Design review of the part built by this model. Coordinates are the model's own, in mm. A direction names the side the tool comes from. Give positions to 0.01 mm unless a question says otherwise; leave off trailing zeros. Loops run counter-clockwise (first coordinate to the right, second up) from the corner with the lowest first, then second, coordinate; pieces in that order, holes last.
from build123d import *

# Parameters (mm, degrees)
SKETCH_1_W          = 106
SKETCH_1_H          = 103
SKETCH_1_W_2        = 102
SKETCH_1_H_2        = 99
EXTRUDE_1_DEPTH     = 25
SKETCH_2_W          = 106
SKETCH_2_H          = 103
EXTRUDE_2_DEPTH     = 1.4
SKETCH_3_R          = 3
SKETCH_3_R_2        = 1.35
EXTRUDE_3_DEPTH     = 5
SKETCH_4_W          = 12.8
SKETCH_4_H          = 11.5
CUT_EXTRUDE_1_DEPTH = 101
FILLET_1_R          = 2
CHAMFER_1_SIZE      = 1
SKETCH_5_R          = 4
SKETCH_5_R_2        = 5
CUT_EXTRUDE_2_DEPTH = 2
SKETCH_6_W          = 3
SKETCH_6_H          = 10
CUT_EXTRUDE_3_DEPTH = 2
SKETCH_8_R          = 1.5
CUT_EXTRUDE_4_DEPTH = 121.470950855
SKETCH_9_R          = 1.5
CUT_EXTRUDE_5_DEPTH = 2
SKETCH_10_W         = 10.5
SKETCH_10_H         = 3
CUT_EXTRUDE_6_DEPTH = 2
SKETCH_11_R         = 6.5
CUT_EXTRUDE_7_DEPTH = 2


with BuildPart() as part:
    # Эскиз1 → Бобышка-Вытянуть1 (new body)
    with BuildSketch(Plane.XY):
        Rectangle(SKETCH_1_W, SKETCH_1_H)
        Rectangle(SKETCH_1_W_2, SKETCH_1_H_2, mode=Mode.SUBTRACT)
    extrude(amount=EXTRUDE_1_DEPTH)

    # Эскиз2 → Бобышка-Вытянуть2 (add)
    with BuildSketch(Plane(origin=(0, 0, 0), x_dir=(-1, 0, 0), z_dir=(0, 0, -1))):
        Rectangle(SKETCH_2_W, SKETCH_2_H)
    extrude(amount=EXTRUDE_2_DEPTH)

    # Эскиз3 → Бобышка-Вытянуть3 (add)
    # profile 1 of 4: a face of its own
    with BuildSketch(Plane.XY):
        with Locations(Location((-45, 39.5, 0), (0, 0, 180))):
            Circle(SKETCH_3_R)
        with Locations((-45, 39.5)):
            Circle(SKETCH_3_R_2, mode=Mode.SUBTRACT)
    # profile 2 of 4: a face of its own
    with BuildSketch(Plane.XY):
        with Locations(Location((45, 39.5, 0), (0, 0, 180))):
            Circle(SKETCH_3_R)
        with Locations((45, 39.5)):
            Circle(SKETCH_3_R_2, mode=Mode.SUBTRACT)
    # profile 3 of 4: a face of its own
    with BuildSketch(Plane.XY):
        with Locations(Location((-45, -43.5, 0), (0, 0, 180))):
            Circle(SKETCH_3_R)
        with Locations((-45, -43.5)):
            Circle(SKETCH_3_R_2, mode=Mode.SUBTRACT)
    # profile 4 of 4: a face of its own
    with BuildSketch(Plane.XY):
        with Locations(Location((45, -43.5, 0), (0, 0, 180))):
            Circle(SKETCH_3_R)
        with Locations((45, -43.5)):
            Circle(SKETCH_3_R_2, mode=Mode.SUBTRACT)
    extrude(amount=EXTRUDE_3_DEPTH)

    # Эскиз4 → Вырез-Вытянуть1 (cut)
    with BuildSketch(Plane.XZ.offset(51.5)):
        with Locations((10.1, 12.35)):
            Rectangle(SKETCH_4_W, SKETCH_4_H)
    extrude(amount=-CUT_EXTRUDE_1_DEPTH, mode=Mode.SUBTRACT)

    # Скругление1
    fillet_1_edges = [part.edges().sort_by_distance(p)[0] for p in [
        (51, -49.5, 12.5),
        (51, 49.5, 12.5),
        (-51, 49.5, 12.5),
        (-51, -49.5, 12.5),
        (53, -51.5, 11.8),
        (-53, -51.5, 11.8),
        (-53, 51.5, 11.8),
        (53, 51.5, 11.8),
    ]]
    fillet(fillet_1_edges, radius=FILLET_1_R)

    # Фаска1
    chamfer_1_edges = [part.edges().sort_by_distance(p)[0] for p in [
        (-51, 0, 0),
        (0, -49.5, 0),
        (51, 0, 0),
        (0, 49.5, 0),
        (50.414213562, -48.914213562, 0),
        (50.414213562, 48.914213562, 0),
        (-50.414213562, 48.914213562, 0),
        (-50.414213562, -48.914213562, 0),
        (-42, 39.5, 0),
        (48, 39.5, 0),
        (-42, -43.5, 0),
        (48, -43.5, 0),
    ]]
    chamfer(chamfer_1_edges, length=CHAMFER_1_SIZE)

    # Эскиз5 → Вырез-Вытянуть2 (cut)
    with BuildSketch(Plane.XZ.offset(51.5)):
        with Locations(Location((32.5, 14.6, 0), (0, 0, 270))):
            Circle(SKETCH_5_R)
        with Locations(Location((-8.3, 14.6, 0), (0, 0, 270))):
            Circle(SKETCH_5_R_2)
    extrude(amount=-CUT_EXTRUDE_2_DEPTH, mode=Mode.SUBTRACT)

    # Эскиз6 → Вырез-Вытянуть3 (cut)
    with BuildSketch(Plane(origin=(53, 0, 0), x_dir=(0, 0, -1), z_dir=(1, 0, 0))):
        with Locations((-23.5, -18.5)):
            Rectangle(SKETCH_6_W, SKETCH_6_H)
        with Locations((-23.5, 7.5)):
            Rectangle(SKETCH_6_W, SKETCH_6_H)
    extrude(amount=-CUT_EXTRUDE_3_DEPTH, mode=Mode.SUBTRACT)

    # Эскиз8 → Вырез-Вытянуть4 (cut, through all)
    with BuildSketch(Plane(origin=(53, 0, 0), x_dir=(0, 0, -1), z_dir=(1, 0, 0))):
        with Locations((-21, 43.5)):
            Circle(SKETCH_8_R)
        with Locations((-21, -43.5)):
            Circle(SKETCH_8_R)
    extrude(amount=-CUT_EXTRUDE_4_DEPTH, mode=Mode.SUBTRACT)

    # Эскиз9 → Вырез-Вытянуть5 (cut)
    with BuildSketch(Plane(origin=(53, 0, 0), x_dir=(0, 0, -1), z_dir=(1, 0, 0))):
        with Locations((-21, -5.5)):
            Circle(SKETCH_9_R)
    extrude(amount=-CUT_EXTRUDE_5_DEPTH, mode=Mode.SUBTRACT)

    # Эскиз10 → Вырез-Вытянуть6 (cut)
    with BuildSketch(Plane(origin=(0, 51.5, 0), x_dir=(1, 0, 0), z_dir=(0, 1, 0))):
        with Locations((9.75, -23.5)):
            Rectangle(SKETCH_10_W, SKETCH_10_H)
    extrude(amount=-CUT_EXTRUDE_6_DEPTH, mode=Mode.SUBTRACT)

    # Эскиз11 → Вырез-Вытянуть7 (cut)
    with BuildSketch(Plane(origin=(53, -1.5, 0), x_dir=(0, 1, 0), z_dir=(-1, 0, 0))):
        with Locations(Location((31, -14.6, 0), (0, 0, 270))):
            Circle(SKETCH_11_R)
    extrude(amount=CUT_EXTRUDE_7_DEPTH, mode=Mode.SUBTRACT)


solid = part.part
Q1. Draft analysis for pull direction X (two halves, no side actions). For faces 4 (the face through (53, -1, 12)), 5 (the face through (-10.215, -50.514, 9.981)), 6 (the face through (1, -51.5, 12)), state which applies: pulls with the +X half, pulls with the -X half, needs draft (parallel to the pull), parting line crosses it, or undercut.
Results:
face 4: pulls with the +X half
face 5: undercut
face 6: needs draft
Q2. Wall thickness on line 1 (Y direction, x = 45, z = 2.3); line 2 (Y direction, x = -14.5, z = 7); line 3 (X direction, y = 11, z = 8): over which ranges is each line inside the solid? List them lowest first.
Results:
line 1: y = -51.5 to -49.5, -46.5 to -44.85, -42.15 to -40.5, 36.5 to 38.15, 40.85 to 42.5, 49.5 to 51.5
line 2: y = -51.5 to -49.5, 49.5 to 51.5
line 3: x = -53 to -51, 51 to 53
Q3. Take a section at B-B (x = 32.5). Give the boundary of the cut face in (y, z).
Results:
outline: (-51.5, -1.4) - (51.5, -1.4) - (51.5, 25) - (49.5, 25) - (49.5, 1) - (48.5, 0) - (-48.5, 0) - (-49.5, 1) - (-49.5, 10.6) - (-51.5, 10.6) - close; (-51.5, 18.6) - (-49.5, 18.6) - (-49.5, 25) - (-51.5, 25) - close
Q4. Tool access review of faces 1 (the face through (-1, -49.5, 13)), 2 (the face through (52.01, -5.43, 22.5)), 3 (the face through (-51.3, 15.5, 25)): name each direction out of +Z, -Z, +X, -X, +Y, -Y from which nothing blocks a thin tool from reaching the whole face with its end or side.
Results:
face 1: +Z
face 2: +X
face 3: +Z, +X, -X, +Y, -Y
Q5. Take a section at A-A (z = 2.5). Give the number of separate pieces and of enclosed holes in the cut face, plus the area to 3 significant figures.
Results:
separate pieces: 5
enclosed holes: 5
area: 910 mm2
Q6. Insertion check: pin 1 (6.5 mm diameter, centred on x = 45, y = 39.5, fed in from +Z); pin 2 (1.6 mm diameter, centred on x = 52, y = -18, fed in from +Z); pin 3 (8 mm diameter, centred on x = -8.3, z = 14.6, fed in from -Y). Each pin has a flat end and moves straight along its axis. Give the tip position at first contact, or say it passes through.
Results:
pin 1: stops at z = 5
pin 2: stops at z = 22
pin 3: stops at y = 49.5
Q7. Take a section at C-C (y = 29.5). Give the boundary of the cut face in (x, z).
Results:
outline: (-53, -1.4) - (53, -1.4) - (53, 8.1) - (51, 8.1) - (51, 1) - (50, 0) - (-50, 0) - (-51, 1) - (-51, 25) - (-53, 25) - close; (51, 21.1) - (53, 21.1) - (53, 25) - (51, 25) - close
